```python
from build123d import *

# Parameters (mm, degrees)
SKETCH1_W           = 18
SKETCH1_H           = 13.1
BOSS_EXTRUDE1_DEPTH = 2
SKETCH2_W           = 3.212723326
SKETCH2_H           = 4.841010911
SKETCH2_W_2         = 6.22211932
SKETCH2_H_2         = 2.776214037
BOSS_EXTRUDE2_DEPTH = 0.5


with BuildPart() as part:
    # Sketch1 → Boss-Extrude1 (new body)
    with BuildSketch(Plane(origin=(0, 0, 0), x_dir=(1, 0, 0), z_dir=(0, 1, 0))):
        with Locations((9, 6.55)):
            Rectangle(SKETCH1_W, SKETCH1_H)
    extrude(amount=BOSS_EXTRUDE1_DEPTH)

    # Sketch2 → Boss-Extrude2 (add)
    with BuildSketch(Plane(origin=(0, 2, 0), x_dir=(1, 0, 0), z_dir=(0, 1, 0))):
        with Locations((4.016157197, 8.925346003)):
            Rectangle(SKETCH2_W, SKETCH2_H)
        with Locations((13.193985763, 4.302170731)):
            Rectangle(SKETCH2_W_2, SKETCH2_H_2)
    extrude(amount=BOSS_EXTRUDE2_DEPTH)


solid = part.part
```
For this review, take the finished solid that the model builds, in its own axes (mm). Coordinates: 2 decimals unless noted, no trailing zeros. Loops run counter-clockwise (first coordinate to the right, second up) from the corner with the lowest first, then second, coordinate; pieces in that order, holes last.
1. For line 1 (Y direction, x = 3.25, z = -3); line 2 (Z direction, x = 3.25, y = 2.25); line 3 (X direction, y = 2.05, z = -11), list the stretches that pass through material, from the lowest coordinate up.
2. Insertion check: P1, Ø3, axis at x = 12, z = -8, coming from the +Y side. The pin has a flat end and moves straight along its axis. Give the tip position at first contact, or say it passes through.
3. Add section D-D, the plane z = -2. Give the boundary of the cut face in (x, y), then the cut area to 3 significant figures.
4. Add section B-B, the plane z = -4.75. Give the boundary of the cut face in (x, y), then the cut area to 3 significant figures.
5. Add section C-C, the plane x = 7.25. Give the boundary of the cut face in (y, z), then the cut area to 3 significant figures.
6. Add section A-A, the plane x = 3.5. Give the boundary of the cut face in (y, z).
Result:
1. line 1: y = 0 to 2
1. line 2: z = -11.35 to -6.5
1. line 3: x = 2.41 to 5.62
2. P1: stops at y = 2
3. outline: (0, 0) - (18, 0) - (18, 2) - (0, 2) - close
3. area: 36.0 mm2
4. outline: (0, 0) - (18, 0) - (18, 2) - (16.31, 2) - (16.31, 2.5) - (10.08, 2.5) - (10.08, 2) - (0, 2) - close
4. area: 39.1 mm2
5. outline: (0, -13.1) - (2, -13.1) - (2, 0) - (0, 0) - close
5. area: 26.2 mm2
6. outline: (0, -13.1) - (2, -13.1) - (2, -11.35) - (2.5, -11.35) - (2.5, -6.5) - (2, -6.5) - (2, 0) - (0, 0) - close
